Verification items for the finished model (mm, model axes). Face numbers are marked on the shaded views. Give positions to 0.01 mm unless a question says otherwise; leave off trailing zeros. Loops run counter-clockwise (first coordinate to the right, second up) from the corner with the lowest first, then second, coordinate; pieces in that order, holes last. Notation, with made-up numbers: M 48,75.5 L 71,75.5 A17 cw 71,99.5 Z; hole C 58,6.5 d4. An arc over 180 degrees is marked long. Write each question's results on one line, items separated by ' | '. Start each with the question number.
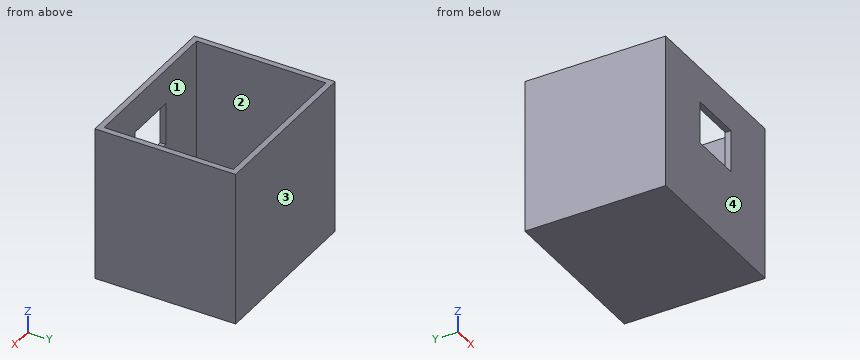
```python
from build123d import *

# Parameters (mm, degrees)
F0_W     = 87.5
F0_H     = 73
F1_DEPTH = 80
F2_T     = -3
F3_W     = 27.5
F3_H     = 22
F4_DEPTH = 3.1


with BuildPart() as f1:
    # F0 (on Top) → F1 (new body)
    with BuildSketch(Plane.XY):
        with Locations((-428.844619, -399.653114)):
            Rectangle(F0_W, F0_H)
    extrude(amount=F1_DEPTH)

    # F2
    f2_openings = [f1.faces().sort_by_distance(p)[0] for p in [
        (-428.844619, -399.653114, 80),
    ]]
    offset(amount=F2_T, openings=f2_openings)

    # F3 (on face) → F4 (cut)
    with BuildSketch(Plane.XZ.offset(436.153114)):
        with Locations((-428.844619, 51)):
            Rectangle(F3_W, F3_H)
    extrude(amount=-F4_DEPTH, mode=Mode.SUBTRACT)


solid = f1.part
```
1. Depth check by flat-ended pin: pin 1 Ø20 at (x, y) = (-434, -404) entering from +Z. Enter the tip coordinate at first touch or a pass-through.
2. Section check C-C, the plane y = -420.5. Record the boundary of the cut face in (x, z).
3. Section check D-D, the plane x = -447.5. Record the boundary of the cut face in (y, z), plus the area to 3 significant figures.
4. Section check A-A, the plane x = -430.5. Record the boundary of the cut face in (y, z), plus the area to 3 significant figures.
5. Section check B-B, the plane z = 34.5. Record the boundary of the cut face in (x, y), plus the area to 3 significant figures.
6. Thickness scan on probe 1 along X at (y, z) = (-424, 61.5); probe 2 along Y at (x, z) = (-412, 44.5); probe 3 along Z at (x, y) = (-398, -381). Record the ranges inside material, lowest first.
7. Release check for a two-part mould opening along Y. For the marked faces 1, 2, 3 and 4 record: released by +Y, released by -Y, zero draft, split by the parting line, or undercut.
Filled sheet:
1) pin 1: z = 3
2) outline: M -472.59,0 L -385.09,0 L -385.09,80 L -388.09,80 L -388.09,3 L -469.59,3 L -469.59,80 L -472.59,80 Z
3) outline: M -436.15,0 L -363.15,0 L -363.15,80 L -366.15,80 L -366.15,3 L -433.15,3 L -433.15,80 L -436.15,80 Z | area: 681 mm2
4) outline: M -436.15,0 L -363.15,0 L -363.15,80 L -366.15,80 L -366.15,3 L -433.15,3 L -433.15,40 L -436.15,40 Z; M -436.15,62 L -433.15,62 L -433.15,80 L -436.15,80 Z | area: 615 mm2
5) outline: M -472.59,-436.15 L -385.09,-436.15 L -385.09,-363.15 L -472.59,-363.15 Z; hole M -469.59,-433.15 L -388.09,-433.15 L -388.09,-366.15 L -469.59,-366.15 Z | area: 927 mm2
6) probe 1: -472.59 to -469.59, -388.09 to -385.09 | probe 2: -436.15 to -433.15, -366.15 to -363.15 | probe 3: 0 to 3
7) face 1: undercut | face 2: undercut | face 3: released by +Y | face 4: released by -Y
